```python
from build123d import *

# Parameters (mm, degrees)
IZIM1_R                     = 1.125
Y_KSEKLIK_EKSTR_ZYON1_DEPTH = 5.5


with BuildPart() as part:
    # Çizim1 → Yükseklik-Ekstrüzyon1 (new body)
    with BuildSketch(Plane.XY):
        with BuildLine():
            Line((-0.73750862, -36.078547579), (0.210244923, -36.078547579))
            Line((0.210244923, -36.078547579), (0.309026113, -39.184890491))
            ThreePointArc((0.309026113, -39.184890491), (0.610430221, -39.4862946), (0.91183433, -39.184890491))
            Line((0.91183433, -39.184890491), (1.002609544, -36.078547579))
            Line((1.002609544, -36.078547579), (1.157998466, -36.078547579))
            Line((1.157998466, -36.078547579), (1.480686358, -36.401235471))
            Line((1.480686358, -36.401235471), (3.507166322, -36.401235471))
            Line((3.507166322, -36.401235471), (3.829854214, -36.078547579))
            Line((3.829854214, -36.078547579), (5.422522789, -36.078547579))
            Line((5.422522789, -36.078547579), (5.526914996, -39.143906466))
            ThreePointArc((5.526914996, -39.143906466), (5.826979248, -39.443970718), (6.1270435, -39.143906466))
            Line((6.1270435, -39.143906466), (6.216621056, -36.078547579))
            Line((6.216621056, -36.078547579), (7.67629389, -36.078547579))
            Line((7.67629389, -36.078547579), (8.097584701, -36.401235471))
            Line((8.097584701, -36.401235471), (8.097584701, -36.457430984))
            Line((8.097584701, -36.457430984), (9.992871432, -36.457430984))
            Line((9.992871432, -36.457430984), (10.371754838, -36.078547579))
            Line((10.371754838, -36.078547579), (10.679552543, -36.078547579))
            Line((10.679552543, -36.078547579), (10.803656958, -39.041199534))
            ThreePointArc((10.803656958, -39.041199534), (11.076182099, -39.313724675), (11.34870724, -39.041199534))
            Line((11.34870724, -39.041199534), (11.469552543, -36.078547579))
            Line((11.469552543, -36.078547579), (12.26249138, -36.078547579))
            Line((12.26249138, -36.078547579), (12.26249138, -29.81509131))
            Line((12.26249138, -29.81509131), (4.18034079, -29.81509131))
            Line((4.18034079, -29.81509131), (4.18034079, -29.31509131))
            ThreePointArc((4.18034079, -29.31509131), (3.624816768, -28.956669378), (3.069292745, -29.31509131))
            Line((3.069292745, -29.31509131), (3.069292745, -29.81509131))
            Line((3.069292745, -29.81509131), (1.165892063, -29.81509131))
            Line((1.165892063, -29.81509131), (1.165892063, -29.744693477))
            ThreePointArc((1.165892063, -29.744693477), (1.184856501, -29.68609964), (1.234556818, -29.649729787))
            Line((1.234556818, -29.649729787), (13.247034334, -25.685962886))
            ThreePointArc((13.247034334, -25.685962886), (13.356857182, -25.468018658), (13.138932408, -25.358157209))
            Line((13.138932408, -25.358157209), (1.064608949, -29.337589121))
            ThreePointArc((1.064608949, -29.337589121), (0.815991055, -29.519422097), (0.721116967, -29.812463042))
            Line((0.721116967, -29.812463042), (0.721116967, -29.81509131))
            Line((0.721116967, -29.81509131), (-0.73750862, -29.81509131))
            Line((-0.73750862, -29.81509131), (-0.73750862, -36.078547579))
        make_face()
        with Locations((2.387599646, -34.883277444)):
            Circle(IZIM1_R, mode=Mode.SUBTRACT)
        with Locations((9.100214646, -34.883277444)):
            Circle(IZIM1_R, mode=Mode.SUBTRACT)
    extrude(amount=Y_KSEKLIK_EKSTR_ZYON1_DEPTH)


solid = part.part
```
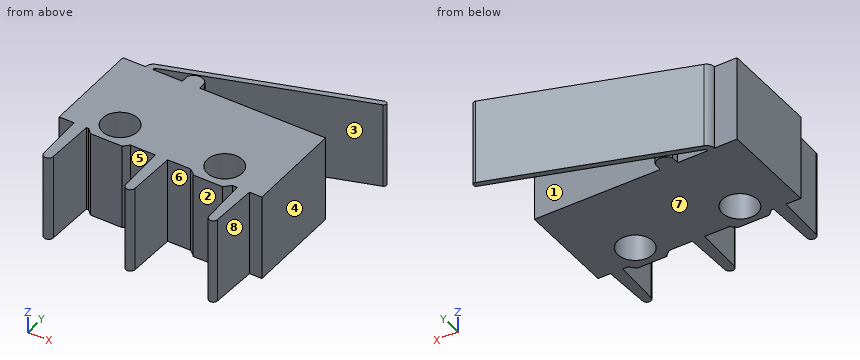
Here's how the part is built. I have some questions about the finished solid (model axes, mm). Face numbers are marked on the shaded views. A direction names the side the tool comes from. Round coordinates to 2 decimals unless told otherwise and drop trailing zeros. Write each loop counter-clockwise with the first axis right and the second up, starting at its lowest first coordinate (ties: lowest second). Pieces come first, ordered by that corner, then holes.
Q1. Please list where these lines run through material, in increasing order: probe 1 along X at (y, z) = (-38, 0.9); probe 2 along Y at (x, z) = (8.5, 1.2); probe 3 along Y at (x, z) = (2.5, 2.6).
Q2. If we section it at D-D on z = 3.3: Give the number of separate pieces and of enclosed holes in the cut face, plus the area to 3 significant figures.
Q3. If we mould it in two halves opening along X, with no side actions, what happens to the marked faces 5, 6, 7 and 8? For each: +X half, -X half, draft (parallel to the pull), parting line (faces both ways), or undercut.
Q4. Which directions (+Z, -Z, +X, -X, +Y, -Y) give clear straight access to the entire face, cutting with the end or side of a thin tool? Please do the marked faces 1, 2, 3 and 4.
Q5. If we section it at B-B on x = 12: Write out the boundary of the cut face in (y, z), plus the area to 3 significant figures.
Q6. If we section it at C-C on x = 2.75: Write out the boundary of the cut face in (y, z).
Q7. If we section it at A-A on y = -34: Write out the boundary of the cut face in (x, z), plus the area to 3 significant figures.
Q8. Will these pins go through, and if not, where does the flat tip stop? P1, Ø0.9, axis at x = 8.5, z = 2, coming from the -Y side; P2, Ø4, axis at x = 9.5, y = -32.5, coming from the -Z side; P3, Ø1, axis at x = 0, z = 4, coming from the -Y side; P4, Ø0.7, axis at x = 7, z = 2, coming from the -Y side.
Answer below:
1. probe 1: x = 0.27 to 0.95, 5.49 to 6.16, 10.76 to 11.39
1. probe 2: y = -36.46 to -35.83, -33.93 to -29.82, -27.25 to -26.89
1. probe 3: y = -36.4 to -36, -33.76 to -29.82, -29.23 to -28.86
2. separate pieces: 1
2. enclosed holes: 2
2. area: 87.2 mm2
3. face 5: undercut
3. face 6: undercut
3. face 7: draft
3. face 8: +X half
4. face 1: +Z, -Z, +X
4. face 2: +Z, -Z, -Y
4. face 3: +Z, -Z
4. face 4: +Z, -Z, +X, -Y
5. outline: (-36.08, 0) - (-29.82, 0) - (-29.82, 5.5) - (-36.08, 5.5) - close; (-26.1, 0) - (-25.73, 0) - (-25.73, 5.5) - (-26.1, 5.5) - close
5. area: 36.5 mm2
6. outline: (-36.4, 0) - (-35.95, 0) - (-35.95, 5.5) - (-36.4, 5.5) - close; (-33.82, 0) - (-29.82, 0) - (-29.82, 5.5) - (-33.82, 5.5) - close; (-29.15, 0) - (-28.78, 0) - (-28.78, 5.5) - (-29.15, 5.5) - close
7. outline: (-0.74, 0) - (1.69, 0) - (1.69, 5.5) - (-0.74, 5.5) - close; (3.08, 0) - (8.4, 0) - (8.4, 5.5) - (3.08, 5.5) - close; (9.8, 0) - (12.26, 0) - (12.26, 5.5) - (9.8, 5.5) - close
7. area: 56.2 mm2
8. P1: stops at y = -36.46
8. P2: stops at z = 0
8. P3: stops at y = -39.47
8. P4: stops at y = -36.08
